```python
from build123d import *

# Parameters (mm, degrees)
P_IDAT_VYSUNUT_M1_DEPTH = 1


with BuildPart() as part:
    # Skica1 → Přidat vysunutím1 (new body)
    with BuildSketch(Plane.XY):
        with BuildLine():
            Line((-50, 16.966408225), (-70, 34.613472684))
            Line((-70, 34.613472684), (-70, 0))
            Line((-70, 0), (-35.640611214, 0))
            Line((-35.640611214, 0), (-14.855667701, -9.644204288))
            Line((-14.855667701, -9.644204288), (30.264283345, -9.644204288))
            Line((30.264283345, -9.644204288), (30, -1.266639703))
            Line((30, -1.266639703), (18, -2.011136657))
            add(Edge.make_bspline(
                [(-50, 16.966408225), (-43.991226664, 11.871570217), (-34.17756419, 5.795583319), (-20.181640748, 0.787148233), (-10.092446875, -1.45782146), (-0.026309786, -2.456617667), (9.343623235, -2.642712691), (15.33383978, -2.176549004), (18, -2.011136657)],
                knots=[0, 0, 0, 0, 0.325390078, 0.471834546, 0.613059233, 0.751676123, 0.88953762, 1, 1, 1, 1], degree=3))
        make_face()
    extrude(amount=P_IDAT_VYSUNUT_M1_DEPTH)


solid = part.part
```
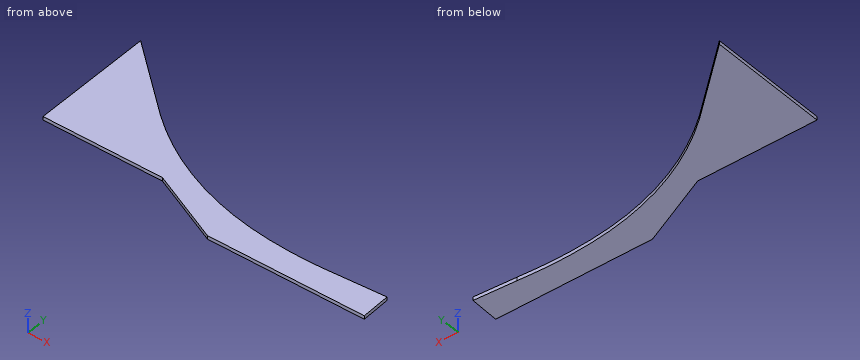
The listing builds one solid part. Answer for the finished solid, in the listing's coordinates (mm). Give positions to 0.01 mm unless a question says otherwise; leave off trailing zeros. Order: outer loops, then holes, each group sorted by start corner. A loop starts at its lowest first (then second) coordinate and runs counter-clockwise, first axis right, second up.
Item 1: The part is cut by section A-A, the plane y = 23.5. Give the vertices of the cut face in (x, z).
From the geometry:
outline: (-70, 0) - (-57.4, 0) - (-57.4, 1) - (-70, 1) - close
Item 2: Find the intervals of material crossed by probe 1 along Y at (x, z) = (-7, 0.2); probe 2 along X at (y, z) = (29, 0.5); probe 3 along X at (y, z) = (-5, 0.7), in increasing order.
From the geometry:
probe 1: y = -9.64 to -1.69
probe 2: x = -70 to -63.64
probe 3: x = -24.86 to 30.12
Item 3: The part is cut by section B-B, the plane y = 30.5. Give the vertices of the cut face in (x, z), and give its area (3 significant figures).
From the geometry:
outline: (-70, 0) - (-65.34, 0) - (-65.34, 1) - (-70, 1) - close
area: 4.66 mm2
